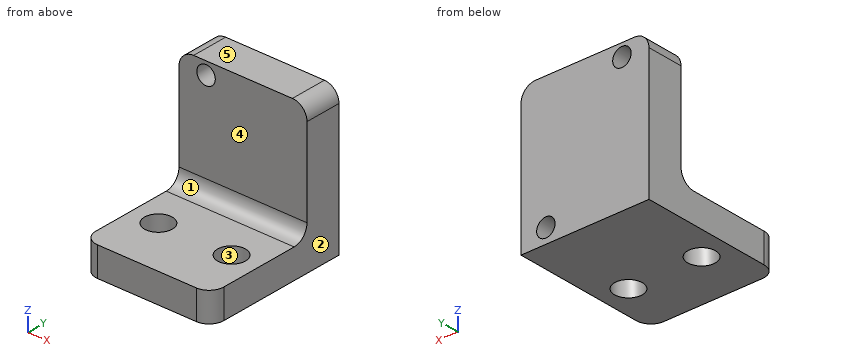
from build123d import *

# Parameters (mm, degrees)
SKETCH1_W           = 22.225
SKETCH1_H           = 25.4
SKETCH1_R           = 1.6002
BOSS_EXTRUDE1_DEPTH = 6.35
SKETCH2_W           = 22.225
SKETCH2_H           = 19.05
SKETCH2_R           = 2.413
BOSS_EXTRUDE2_DEPTH = 5.08
FILLET1_R           = 2.54


with BuildPart() as part:
    # Sketch1 → Boss-Extrude1 (new body)
    with BuildSketch(Plane(origin=(0, 0, 0), x_dir=(1, 0, 0), z_dir=(0, 1, 0))):
        with Locations((3.3655, 0)):
            Rectangle(SKETCH1_W, SKETCH1_H)
        with Locations(Location((10.16, 10.16, 0), (0, 0, 270))):
            Circle(SKETCH1_R, mode=Mode.SUBTRACT)
        with Locations(Location((-3.044225571, -10.529380079, 0), (0, 0, 270))):
            Circle(SKETCH1_R, mode=Mode.SUBTRACT)
    extrude(amount=-BOSS_EXTRUDE1_DEPTH)

    # Sketch2 → Boss-Extrude2 (add)
    with BuildSketch(Plane(origin=(0, 0, -12.7), x_dir=(-1, 0, 0), z_dir=(0, 0, -1))):
        with Locations((-3.3655, -15.875)):
            Rectangle(SKETCH2_W, SKETCH2_H)
        with Locations((-9.7155, -15.875)):
            Circle(SKETCH2_R, mode=Mode.SUBTRACT)
        with Locations((2.9845, -15.875)):
            Circle(SKETCH2_R, mode=Mode.SUBTRACT)
    extrude(amount=-BOSS_EXTRUDE2_DEPTH)

    # Fillet1
    fillet1_edges = [part.edges().sort_by_distance(p)[0] for p in [
        (3.3655, -6.35, -7.62),
        (14.478, -25.4, -10.16),
        (-7.747, -25.4, -10.16),
        (14.478, -3.175, 12.7),
        (-7.747, -3.175, 12.7),
    ]]
    fillet(fillet1_edges, radius=FILLET1_R)


solid = part.part
Build history of the part. All positions in model axes, mm. Face numbers are marked on the shaded views. A direction names the side the tool comes from. Give positions to 0.01 mm unless a question says otherwise; leave off trailing zeros. Loops run counter-clockwise (first coordinate to the right, second up) from the corner with the lowest first, then second, coordinate; pieces in that order, holes last. Notation, with made-up numbers: (-16, 74) - (3, 74) arc R27 ccw to (3, 92) - close; hole circle Ø4 at (74.5, -1). An arc over 180 degrees is marked (long way). Write item = value, one per line. Start each with the question number.
1) Pull direction Y, two halves, no side cores. Call the marked faces 1, 2 and 3: +Y half, -Y half, draft (parallel to the pull), parting line (faces both ways), or undercut.
2) Band-saw the part on D-D on z = 1.25. Give the cut face in (x, y).
3) Band-saw the part on A-A on x = 11. Give the cut face in (y, z).
4) Probe probe 1 along X at (y, z) = (-3.5, -10.16); probe 2 along X at (y, z) = (-17.5, -8.75); probe 3 along Z at (x, y) = (9.75, -13.25). List the from-to ranges inside material, lowest first. Write a range as from..to.
5) Band-saw the part on C-C on x = 1.75. Give the cut face in (y, z).
6) Drop flat-ended pins along their axis: pin 1 Ø8.5 at (x, y) = (7.5, -17.5) entering from +Z; pin 2 Ø9 at (x, z) = (1.5, 4.5) entering from -Y; pin 3 Ø1.6 at (x, z) = (10, -10.5) entering from +Y; pin 4 Ø4 at (x, y) = (-2.98, -15.88) entering from +Z. Give the stop position or say it passes through.
7) Band-saw the part on B-B on z = -10.5. Count the separate pieces of the cut face and the enclosed holes in it, plus the area to 3 significant figures.
8) Tool access for the marked faces 4 and 5: list every direction of +Z, -Z, +X, -X, +Y, -Y with a clear straight run to the whole face (end or side of a thin tool).
Final values:
q1.face_1 = -Y half
q1.face_2 = draft
q1.face_3 = undercut
q2.outline = (-7.75, -6.35) - (14.48, -6.35) - (14.48, 0) - (-7.75, 0) - close
q3.outline = (-25.4, -12.7) - (-17.92, -12.7) - (-17.92, -7.62) - (-25.4, -7.62) - close; (-13.83, -12.7) - (0, -12.7) - (0, -11.52) - (-6.35, -11.52) - (-6.35, -8.8) - (0, -8.8) - (0, 12.7) - (-6.35, 12.7) - (-6.35, -5.08) arc R2.54 cw to (-8.89, -7.62) - (-13.83, -7.62) - close
q4.probe_1 = -7.75..8.56, 11.76..14.48
q4.probe_2 = -7.75..-4.77, -1.2..7.93, 11.5..14.48
q4.probe_3 = -12.7..-7.62
q5.outline = (-25.4, -12.7) - (0, -12.7) - (0, 12.7) - (-6.35, 12.7) - (-6.35, -5.08) arc R2.54 cw to (-8.89, -7.62) - (-25.4, -7.62) - close
q6.pin_1 = -7.62
q6.pin_2 = -6.35
q6.pin_3 = -6.35
q6.pin_4 = through
q7.separate_pieces = 1
q7.enclosed_holes = 2
q7.area = 505 mm²
q8.face_4 = +Z, +X, -X, -Y
q8.face_5 = +Z, +X, -X, +Y, -Y
